Could you check a few things on this model? Use its own coordinates, in mm. Coordinates: 2 decimals unless noted, no trailing zeros. Order: outer loops, then holes, each group sorted by start corner. A loop starts at its lowest first (then second) coordinate and runs counter-clockwise, first axis right, second up. Notation, with made-up numbers: (-4.5, -39.5) -> (15.5, -39.5) arc R21 ccw to (15.5, -11.5) -> close; hole circle Ø5 at (89, 60). An arc over 180 degrees is marked (long way). Use a Markdown table: item, result. Add a question column.
1) If we section it at A-A (z = -450): Write out the boundary of the cut face in (x, y), plus the area to 3 significant figures.
2) If we section it at C-C (y = -70): Write out the boundary of the cut face in (x, z), plus the area to 3 significant figures.
3) If we section it at D-D (z = -269): Write out the boundary of the cut face in (x, y), plus the area to 3 significant figures.
4) Will these pins go through, and if not, where does the flat tip stop? pin 1 Ø3 at (x, z) = (0.5, -302) entering from +Y; pin 2 Ø3 at (x, z) = (2.5, -140.5) entering from -Y; pin 3 Ø2 at (x, y) = (-2, 41.5) entering from +Z.
5) If we section it at B-B (x = -2.25): Write out the boundary of the cut face in (y, z).
6) If I drill on L1, parallel to Y at x = -1.5, z = -399; L2, parallel to Z at x = 0.75, y = -8; L3, parallel to Y at x = -2, z = -408.5, over which ranges is the centre line in solid material (lowest first)? Write a range as [from, to].
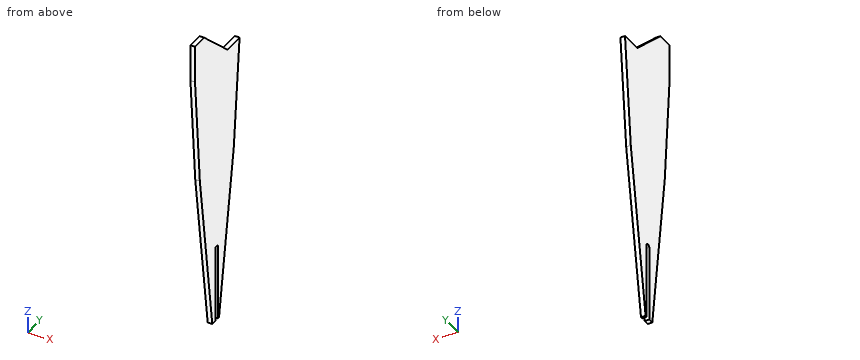
```python
from build123d import *

# Parameters (mm, degrees)
BOSS_EXTRUDE1_DEPTH      = 4.3
BOSS_EXTRUDE1_DEPTH_BACK = 4.3
SKETCH3_W                = 152
SKETCH3_H                = 8.6
CUT_EXTRUDE1_DEPTH       = 520.595708462
FILLET1_R                = 3


with BuildPart() as part:
    # Sketch2 → Boss-Extrude1 (new, two sides: drawn at the far end of the back side and taken through both)
    with BuildSketch(Plane(origin=(0, 0, 0), x_dir=(0, 0, -1), z_dir=(1, 0, 0)).offset(-BOSS_EXTRUDE1_DEPTH_BACK)):
        Polygon((0, 67.22485033), (205.165503831, 48.288859026), (513.4, -0.530689138), (513.4, -22.650154351), (205.250409944, -63.717607751), (0, -79.537288439), (-70, -79.537288439), (-70, -49.537288439), (0, 27.22485033), align=None)
    extrude(amount=BOSS_EXTRUDE1_DEPTH + BOSS_EXTRUDE1_DEPTH_BACK)

    # Sketch3 → Cut-Extrude1 (cut, through all)
    with BuildSketch(Plane(origin=(4.3, 0, 0), x_dir=(0, 0, -1), z_dir=(1, 0, 0))):
        with Locations((443.4, -8.3)):
            Rectangle(SKETCH3_W, SKETCH3_H)
    extrude(amount=-CUT_EXTRUDE1_DEPTH, mode=Mode.SUBTRACT)

    # Fillet1
    fillet1_edges = [part.edges().sort_by_distance(p)[0] for p in [
        (0, -12.6, -367.4),
        (0, -4, -367.4),
    ]]
    fillet(fillet1_edges, radius=FILLET1_R)


solid = part.part
```
Answer sheet:
| question | item | result |
|---|---|---|
| 1 | outline | (-4.3, -31.1) -> (4.3, -31.1) -> (4.3, -12.6) -> (-4.3, -12.6) -> close; (-4.3, -4) -> (4.3, -4) -> (4.3, 9.51) -> (-4.3, 9.51) -> close |
| 1 | area | 275 mm2 |
| 2 | outline | (-4.3, -123.74) -> (4.3, -123.74) -> (4.3, 70) -> (-4.3, 70) -> close |
| 2 | area | 1,670 mm2 |
| 3 | outline | (-4.3, -55.22) -> (4.3, -55.22) -> (4.3, 38.18) -> (-4.3, 38.18) -> close |
| 3 | area | 803 mm2 |
| 4 | pin 1 | y = 33.19 |
| 4 | pin 2 | y = -68.82 |
| 4 | pin 3 | z = 0 |
| 5 | outline | (-79.54, 0) -> (-63.72, -205.25) -> (-22.65, -513.4) -> (-12.6, -513.4) -> (-12.6, -370.4) arc R3 cw to (-9.6, -367.4) -> (-7, -367.4) arc R3 cw to (-4, -370.4) -> (-4, -513.4) -> (-0.53, -513.4) -> (48.29, -205.17) -> (67.22, 0) -> (27.22, 0) -> (-49.54, 70) -> (-79.54, 70) -> close |
| 6 | L1 | [-37.9, -12.6], [-4, 17.59] |
| 6 | L2 | [-367.4, 32.12] |
| 6 | L3 | [-36.63, -12.6], [-4, 16.08] |
